```python
from build123d import *

# Parameters (mm, degrees)
CROQUIS1_W              = 25.4
CROQUIS1_H              = 12.7
SALIENTE_EXTRUIR1_DEPTH = 40
CROQUIS2_W              = 40.869814695
CROQUIS2_H              = 51.393723527
CORTAR_EXTRUIR1_DEPTH   = 30
CROQUIS3_R              = 2.5
CORTAR_EXTRUIR2_DEPTH   = 30
CROQUIS4_R              = 2.5
CORTAR_EXTRUIR3_DEPTH   = 30


with BuildPart() as part:
    # Croquis1 → Saliente-Extruir1 (new body)
    with BuildSketch(Plane.XY):
        with Locations((12.7, 6.35)):
            Rectangle(CROQUIS1_W, CROQUIS1_H)
    extrude(amount=SALIENTE_EXTRUIR1_DEPTH)

    # Croquis2 → Cortar-Extruir1 (cut)
    with BuildSketch(Plane(origin=(0, 12.7, 0), x_dir=(1, 0, 0), z_dir=(0, 1, 0))):
        with Locations((12.097003992, -18.212370052)):
            Rectangle(CROQUIS2_W, CROQUIS2_H)
        with BuildLine():
            Line((25.4, 0), (3, 0))
            ThreePointArc((3, 0), (0.878679656, -0.878679656), (0, -3))
            Line((0, -3), (0, -25.4))
            Line((0, -25.4), (3, -25.4))
            Line((3, -25.4), (3, -3))
            Line((3, -3), (25.4, -3))
            Line((25.4, -3), (25.4, 0))
        make_face(mode=Mode.SUBTRACT)
    extrude(amount=-CORTAR_EXTRUIR1_DEPTH, mode=Mode.SUBTRACT)

    # Croquis3 → Cortar-Extruir2 (cut)
    with BuildSketch(Plane(origin=(3, 0, 0), x_dir=(0, 0, -1), z_dir=(1, 0, 0))):
        with Locations((-20.4, 6.35)):
            Circle(CROQUIS3_R)
    extrude(amount=-CORTAR_EXTRUIR2_DEPTH, mode=Mode.SUBTRACT)

    # Croquis4 → Cortar-Extruir3 (cut)
    with BuildSketch(Plane.XY.offset(3)):
        with Locations((20.4, 6.35)):
            Circle(CROQUIS4_R)
    extrude(amount=-CORTAR_EXTRUIR3_DEPTH, mode=Mode.SUBTRACT)


solid = part.part
```
Work out the finished part from the listing and answer in its coordinate system (mm). A direction names the side the tool comes from. Round coordinates to 2 decimals unless told otherwise and drop trailing zeros. Loops run counter-clockwise (first coordinate to the right, second up) from the corner with the lowest first, then second, coordinate; pieces in that order, holes last. Notation, with made-up numbers: M 81.25,-10.75 L 89.25,-10.75 A16 ccw 89.25,5.25 Z; hole C 25.25,17 d7. An arc over 180 degrees is marked long. One line per question, with ' | ' between items.
Q1. The mould has two halves that part along Z. Classify faces 3 (the flat face through (1, 6, 25.4)), 4 (the cylindrical face through (22.785, 7.101, 1.521)), 5 (the cylindrical face through (1.52, 8.04, 22.24)): +Z half, -Z half, draft (parallel to the pull), parting line (faces both ways), or undercut.
Conclusion:
face 3: +Z half | face 4: draft | face 5: undercut
Q2. A tool of negligible diameter and unlimited length cuts with its end or side. For faces 1 (the flat face through (14, 6, 3)), 2 (the flat face through (2, 0, 7)), from which of +Z, -Z, +X, -X, +Y, -Y can it reach the whole face along a straight path? Write none if from no direction.
Conclusion:
face 1: +Z, +X, +Y, -Y | face 2: +Z, -Z, +X, -X, -Y
Q3. Find section B-B, the plane x = 20.4. Give the vertices of the cut face in (y, z), then the cut area to 3 significant figures.
Conclusion:
outline: M 0,0 L 3.85,0 L 3.85,3 L 0,3 Z; M 8.85,0 L 12.7,0 L 12.7,3 L 8.85,3 Z | area: 23.1 mm2
Q4. Find section A-A, the plane y = 6.35. Give the vertices of the cut face in (x, z).
Conclusion:
outline: M 0,3 A3 ccw 3,0 L 17.9,0 L 17.9,3 L 3,3 L 3,17.9 L 0,17.9 Z; M 0,22.9 L 3,22.9 L 3,25.4 L 0,25.4 Z; M 22.9,0 L 25.4,0 L 25.4,3 L 22.9,3 Z
Q5. Find section C-C, the plane z = 20.4. Give the vertices of the cut face in (x, y).
Conclusion:
outline: M 0,0 L 3,0 L 3,3.85 L 0,3.85 Z; M 0,8.85 L 3,8.85 L 3,12.7 L 0,12.7 Z
Q6. Find section D-D, the plane y = 3. Give the vertices of the cut face in (x, z), then the cut area to 3 significant figures.
Conclusion:
outline: M 0,3 A3 ccw 3,0 L 25.4,0 L 25.4,3 L 3,3 L 3,25.4 L 0,25.4 Z | area: 141 mm2
Q7. Consider line 1 along Y through (x, z) = (20.4, 1.9); line 2 along X through (y, z) = (2.5, 13). Determine where each line is inside the solid, lowest interval first. Write a range as from..to.
Conclusion:
line 1: y = 0..3.85, 8.85..12.7 | line 2: x = 0..3
Q8. Each of these flat-tipped pins is pushed along its axis until it touches: pin 1 Ø1.5 at (y, z) = (2, 20.5) entering from +X; pin 2 Ø1.5 at (x, y) = (12, 3) entering from +Z. Where does it stop, or does it pass through?
Conclusion:
pin 1: stops at x = 3 | pin 2: stops at z = 3
